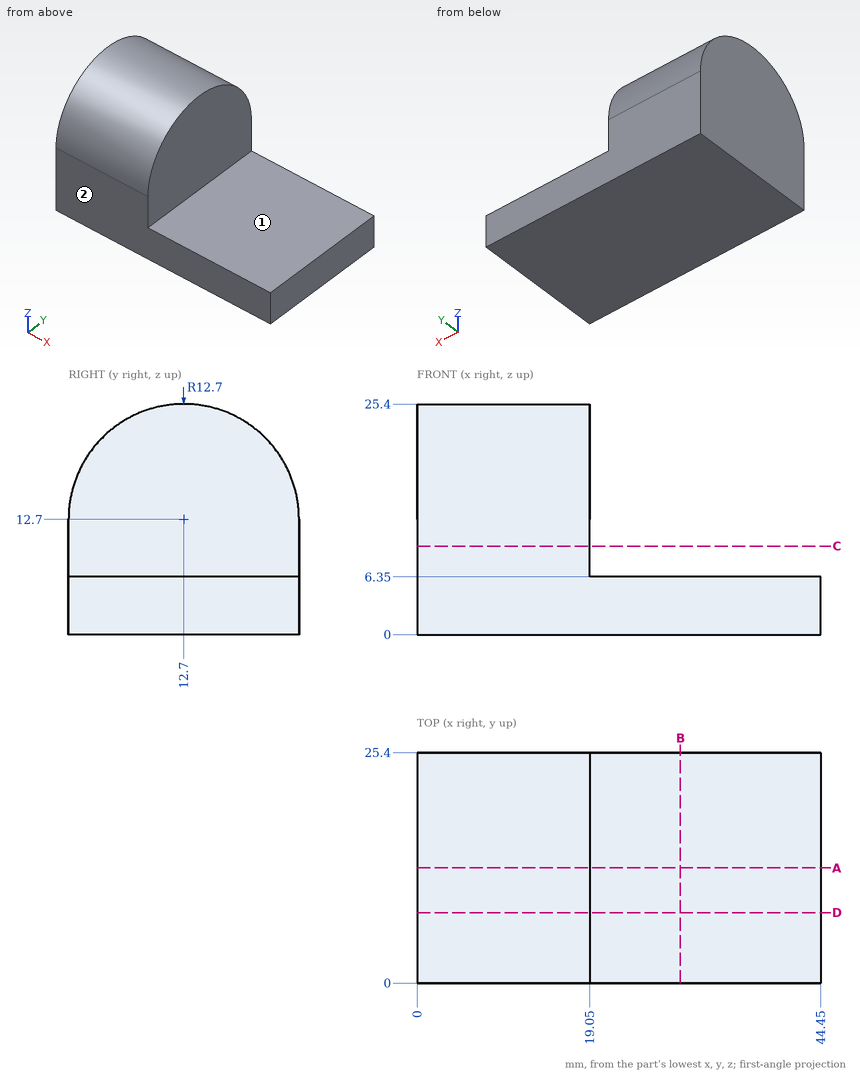
Verification items for this drawing (mm, ordinates from the low corner). A direction names the side the tool comes from. Round coordinates to 2 decimals unless told otherwise and drop trailing zeros. Loops run counter-clockwise (first coordinate to the right, second up) from the corner with the lowest first, then second, coordinate; pieces in that order, holes last. Notation, with made-up numbers: (1.5, 18.25) -> (37.5, 18.25) arc R27 ccw to (37.5, 34.25) -> close; hole circle Ø11 at (7, 16.25). An arc over 180 degrees is marked (long way). Write item = value, one per line. Start each with the question number.
1) Sectioned sample at C-C, the plane z = 9.75. Record the cut outline in (x, y).
2) Sectioned sample at B-B, the plane x = 29. Record the cut outline in (y, z), plus the area to 3 significant figures.
3) Gauge pin test, flat ends, axial feed: pin 1 Ø2 at (x, z) = (19, 17) entering from -Y; pin 2 Ø7.5 at (x, y) = (31, 12.5) entering from +Z; pin 3 Ø15 at (y, z) = (13, 17.5) entering from +X. Record the tip position at first contact, or that the pin passes through.
4) Thickness scan on probe 1 along X at (y, z) = (21, 14.5); probe 2 along Z at (x, y) = (25, 2); probe 3 along Z at (x, y) = (11.5, 24.25). Record the ranges inside material, lowest first.
5) Sectioned sample at A-A, the plane y = 12.7. Record the cut outline in (x, z).
6) Set-up check for the marked faces 1 and 2: record each of +Z, -Z, +X, -X, +Y, -Y from which the full face is reachable in a straight line by a thin tool's end or side.
7) Sectioned sample at D-D, the plane y = 7.75. Record the cut outline in (x, z).
Results are:
q1.outline = (0, 0) -> (19.05, 0) -> (19.05, 25.4) -> (0, 25.4) -> close
q2.outline = (0, 0) -> (25.4, 0) -> (25.4, 6.35) -> (0, 6.35) -> close
q2.area = 161 mm^2
q3.pin_1 = 0.44
q3.pin_2 = 6.35
q3.pin_3 = 19.05
q4.probe_1 = 0 to 19.05
q4.probe_2 = 0 to 6.35
q4.probe_3 = 0 to 17.98
q5.outline = (0, 0) -> (44.45, 0) -> (44.45, 6.35) -> (19.05, 6.35) -> (19.05, 25.4) -> (0, 25.4) -> close
q6.face_1 = +Z, +X, +Y, -Y
q6.face_2 = +Z, -Z, +X, -X, -Y
q7.outline = (0, 0) -> (44.45, 0) -> (44.45, 6.35) -> (19.05, 6.35) -> (19.05, 24.4) -> (0, 24.4) -> close
